Autodesk Inventor part; units mm, degrees
ref_plane "YZ Plane" through (0, 0, 0) normal (1, 0, 0) x (0, 1, 0)
ref_plane "XZ Plane" through (0, 0, 0) normal (0, 1, 0) x (-1, 0, 0)
ref_plane "XY Plane" through (0, 0, 0) normal (0, 0, 1) x (1, 0, 0)
sketch "スケッチ1" plane through (0, 0, 0) normal (0, 1, 0) x (-1, 0, 0)
  line L0 (0, 0) -> (310, 0)
  line L1 (310, 0) -> (310, -235)
  line L2 (310, -235) -> (0, -235)
  line L3 (0, -235) -> (0, 0)
  dimension "d0" = 310
  dimension "d1" = 235
extrude "押し出し1" add sketch "スケッチ1" along normal blind 3
sketch "スケッチ2" plane through (0, 3, 0) normal (0, 1, 0) x (1, 0, 0)
  line L0 (-155, -40) -> (-155, 284.5269)
  line L1 (-155, 284.5269) -> (-194.2717, 284.5269)
  line L2 (30, 117.5) -> (-350, 117.5)
  line L3 (0, 0) -> (0, 235)
  line L4 (-310, 0) -> (0, 0)
  circle A0 centre (-195, 10) radius 5
  circle A1 centre (-115, 10) radius 5
  circle A2 centre (-195, 225) radius 5
  circle A3 centre (-115, 225) radius 5
  circle A4 centre (-195, 50) radius 5
  circle A5 centre (-115, 50) radius 5
  circle A6 centre (-195, 185) radius 5
  circle A7 centre (-115, 185) radius 5
  circle A8 centre (-295, 157.5) radius 5
  line L5 (-310, 235) -> (-310, 0)
  circle A9 centre (-295, 77.5) radius 5
  circle A10 centre (-15, 157.5) radius 5
  circle A11 centre (-15, 77.5) radius 5
  circle A12 centre (-255, 157.5) radius 5
  circle A13 centre (-255, 77.5) radius 5
  circle A14 centre (-55, 157.5) radius 5
  circle A15 centre (-55, 77.5) radius 5
  dimension "d4" = 155
  dimension "d5" = 117.5
  dimension "d6" = 10
  dimension "d7" = 40
  dimension "d8" = 10
  dimension "d9" = 10
  dimension "d10" = 40
  dimension "d11" = 10
  dimension "d12" = 15
  dimension "d13" = 40
  dimension "d14" = 10
  dimension "d15" = 40
extrude "押し出し2" cut sketch "スケッチ2" against normal blind 3 contours A0 | A1 | A2 | A3 | A4 | A5 | A6 | A7 | A8 | A9 | A10 | A11 | A12 | A13 | A14 | A15
properties part number "base_diff_02" material "アルミニウム 6061"
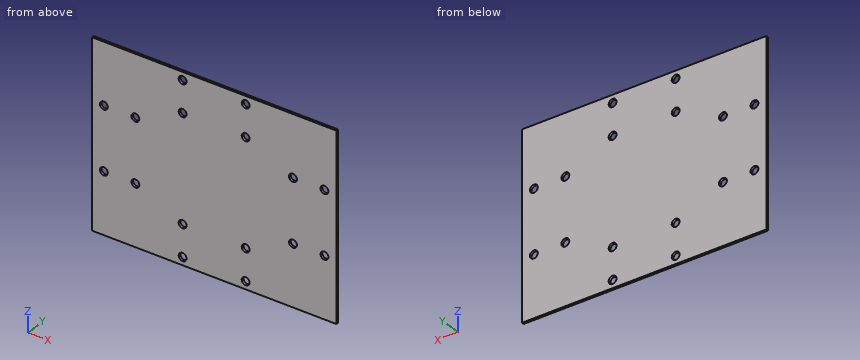
Model file for the job. Use its own axes, mm. Give positions to 0.01 mm unless a question says otherwise; leave off trailing zeros. Write each loop counter-clockwise with the first axis right and the second up, starting at its lowest first coordinate (ties: lowest second). Pieces come first, ordered by that corner, then holes. Notation, with made-up numbers: M -9.5,-16 L 35.5,-16 A32 cw 35.5,12 Z; hole C -24.5,12 d2. An arc over 180 degrees is marked long. One line per item, written item: value. Start each with the question number.
Q1. Saw through at A-A, the plane x = -15. Write the cut outline in (y, z), plus the area to 3 significant figures.
Q2. Probe probe 1 along X at (y, z) = (0.95, -157.5); probe 2 along Z at (x, y) = (-255, 1); probe 3 along Z at (x, y) = (-195, 0.6). List the from-to ranges inside material, lowest first. Write a range as [from, to].
Q3. Saw through at C-C, the plane z = -157.5. Write the cut outline in (x, y).
Q4. Saw through at B-B, the plane z = -10. Write the cut outline in (x, y).
Q5. Saw through at D-D, the plane y = 1.15. State how many separate pieces and enclosed holes the cut face has, plus the area to 3 significant figures.
Output values:
1. outline: M 0,-235 L 3,-235 L 3,-162.5 L 0,-162.5 Z; M 0,-152.5 L 3,-152.5 L 3,-82.5 L 0,-82.5 Z; M 0,-72.5 L 3,-72.5 L 3,0 L 0,0 Z
1. area: 645 mm²
2. probe 1: x = [-310, -300], [-290, -260], [-250, -60], [-50, -20], [-10, 0]
2. probe 2: z = [-235, -162.5], [-152.5, -82.5], [-72.5, 0]
2. probe 3: z = [-235, -230], [-220, -190], [-180, -55], [-45, -15], [-5, 0]
3. outline: M -310,0 L -300,0 L -300,3 L -310,3 Z; M -290,0 L -260,0 L -260,3 L -290,3 Z; M -250,0 L -60,0 L -60,3 L -250,3 Z; M -50,0 L -20,0 L -20,3 L -50,3 Z; M -10,0 L 0,0 L 0,3 L -10,3 Z
4. outline: M -310,0 L -200,0 L -200,3 L -310,3 Z; M -190,0 L -120,0 L -120,3 L -190,3 Z; M -110,0 L 0,0 L 0,3 L -110,3 Z
5. separate pieces: 1
5. enclosed holes: 16
5. area: 71,600 mm²
